Autodesk Fusion 360 part; units mm, degrees
sketch "Sketch1" plane through (0, 0, 0) normal (0, 0, 1) x (1, 0, 0)
  circle A0 centre (0, 11) radius 32.5228
  circle A1 centre (0, 11) radius 35.5057
  line L0 (27.2057, -11.8146) -> (27.2057, -45)
  line L1 (27.2057, -45) -> (16.1805, -20.6046)
  line L2 (24.1506, -15.027) -> (24.1506, -30)
  line L3 (24.1506, -30) -> (19.1372, -18.9069)
  line L4 (-16.1421, -20.6242) -> (-27.4351, -45.7523)
  line L5 (-27.4351, -45.7523) -> (-27.4351, 28.4657)
  line L6 (27.4351, 28.4657) -> (27.2057, -45)
  line L7 (24.15, 23.7181) -> (24.1506, -30)
  line L8 (24.15, 23.7181) -> (3.6905, -21.3128)
  line L9 (-3.6905, -21.3128) -> (-24.2501, 23.7181)
  line L10 (-24.2501, 23.7181) -> (-24.2495, -31.0996)
  line L11 (-24.2495, -31.0996) -> (-18.8513, -19.088)
  line L12 (0, -21.5228) -> (24.3204, 32.5929)
  line L13 (0, -21.5228) -> (-24.5749, 32.3028)
  line L14 (23.0617, -11.9324) -> (-23.0612, -11.9329)
  line L15 (26.1993, -8.27) -> (-24.2497, -8.2706)
  line L16 (-5, 44) -> (6, 44)
  line L17 (6, 44) -> (6, 51)
  line L18 (6, 51) -> (-5, 51)
  line L19 (-5, 51) -> (-5, 44)
  line L20 (4, 49) -> (-3, 49)
  line L21 (-3, 49) -> (-3, 46.3788)
  line L22 (-3, 46.3788) -> (4, 46.3788)
  line L23 (4, 46.3788) -> (4, 49)
  dimension "d3" = 7
extrude "Extrude1" add sketch "Sketch1" along normal blind 5 contours A0 A1 L5 L6 L16 L17 L19 | A0 L6 L7 L8 L12 L15 | A0 A1 L6 L7 | A0 L7 L15 | A0 L5 L9 L10 L13 L15 | L8 L12 L14 L15 | L12 L13 L14 L15 | A0 A1 L7 L10 | A0 L7 L8 L14 L15 | A1 L0 L1 L2 L3 L7 | L9 L13 L14 L15 | A0 L8 L12 L14 | A1 L16 L17 L19 L22 | A0 A1 L5 L10 | A0 L9 L13 L14 | A0 L9 L10 L14 L15 | A1 L22 | A1 L4 L5 L10 L11
extrude "Extrude2" add sketch "Sketch1" along normal blind 5 contours A1 L16 L17 L19 L22 | A1 L17 L18 L19 L20 L21 L22 L23
Check sheet for the modelled part. Datum: model origin and axes. Units: mm. A direction names the side the tool comes from. Give positions to 0.01 mm unless a question says otherwise; leave off trailing zeros. Loops run counter-clockwise (first coordinate to the right, second up) from the corner with the lowest first, then second, coordinate; pieces in that order, holes last. Notation, with made-up numbers: M 10,-24.75 L 41,-24.75 A23 cw 41,-7.75 Z; hole C 21,63.25 d5. An arc over 180 degrees is marked long. Answer as a JSON object with one key per item and string values. Group by question number.
Q1. Go/stop test with flat-tipped pins: P1, Ø1, axis at x = 8, z = 3, coming from the +Y side; P2, Ø2.5, axis at y = 47.5, z = 3.5, coming from the -X side; P3, Ø1.5, axis at y = -21.5, z = 3.5, coming from the -X side. Record where each tip stops, or that it passes through.
Q2. Cross-section at B-B on x = -28.5. Record the cut outline in (y, z).
Q3. Cross-section at D-D on x = 20.5. Record the cut outline in (y, z), then the cut area to 3 significant figures.
Q4. Release check for a two-part mould opening along X. For faces 1 (the cylindrical face through (21.77, -17.05, 2.46)), 2 (the flat face through (27.206, -28, 2)), 3 (the cylindrical face through (-0.58, 43.518, 2.465)), 4 (the flat face through (-8.1, -4.3, 0)) record: released by +X, released by -X, zero draft, split by the parting line, or undercut.
Q5. Material ranges on line 1 along X through (y, z) = (0, 3.25); line 2 along Y through (x, z) = (-19.5, 0.35); line 3 along Y through (x, z) = (-17, 1), recorded low to high. Write a range as [from, to].
Q6. Cross-section at A-A on y = 22. Record the cut outline in (x, z).
Q7. Cross-section at C-C on x = -1. Record the cut outline in (y, z), then the cut area to 3 significant figures.
Q8. Access from +Z, -Z, +X, -X, +Y, -Y to the whole of each face (thin tool, end or side, straight path). Record for faces 5 (the flat face through (-2.16, -16.79, 2.46)), 6 (the flat face through (-8.1, -4.3, 5)).
Evaluation:
{
 "1": {"P1": "stops at y = 45.7", "P2": "stops at x = -5", "P3": "stops at x = -27.44"},
 "2": {"outline": "M -10.18,0 L -4.67,0 L -4.67,5 L -10.18,5 Z; M 26.67,0 L 32.18,0 L 32.18,5 L 26.67,5 Z"},
 "3": {"outline": "M -30.16,0 L -21.92,0 L -21.92,5 L -30.16,5 Z; M -17.99,0 L -14.25,0 L -14.25,5 L -17.99,5 Z; M -11.93,0 L -8.27,0 L -8.27,5 L -11.93,5 Z; M 15.68,0 L 24.09,0 L 24.09,5 L 15.68,5 Z; M 36.25,0 L 39.99,0 L 39.99,5 L 36.25,5 Z", "area": "139 mm2"},
 "4": {"face 1": "undercut", "face 2": "released by +X", "face 3": "undercut", "face 4": "zero draft"},
 "5": {"line 1": "x = [-33.76, -30.61], [-27.44, -24.25], [-13.42, -9.83], [9.67, 13.37], [24.15, 27.35], [30.61, 33.76]", "line 2": "y = [-28.1, -20.53], [-18.67, -15.03], [-11.93, -8.27], [13.31, 21.19], [37.03, 40.67]", "line 3": "y = [-22.53, -16.73], [-11.93, -8.27], [7.84, 15.71], [38.73, 42.17]"},
 "6": {"outline": "M -33.76,0 L -30.61,0 L -30.61,5 L -33.76,5 Z; M -27.44,0 L -24.25,0 L -24.25,5 L -27.44,5 Z; M -23.47,0 L -19.87,0 L -19.87,5 L -23.47,5 Z; M 19.56,0 L 23.37,0 L 23.37,5 L 19.56,5 Z; M 24.15,0 L 27.41,0 L 27.41,5 L 24.15,5 Z; M 30.61,0 L 33.76,0 L 33.76,5 L 30.61,5 Z"},
 "7": {"outline": "M -24.49,0 L -19.33,0 L -19.33,5 L -24.49,5 Z; M -11.93,0 L -8.27,0 L -8.27,5 L -11.93,5 Z; M 43.51,0 L 46.49,0 L 46.49,5 L 43.51,5 Z; M 49,0 L 51,0 L 51,5 L 49,5 Z", "area": "69.0 mm2"},
 "8": {"face 5": "+Z, -Z", "face 6": "+Z, +X, -X, +Y, -Y"}
}
